Model file for the job. Use its own axes, mm. Round coordinates to 2 decimals unless told otherwise and drop trailing zeros. Loops run counter-clockwise (first coordinate to the right, second up) from the corner with the lowest first, then second, coordinate; pieces in that order, holes last. Notation, with made-up numbers: M -37.5,2 L -31.5,2 A26 ccw -31.5,20 Z; hole C 80,28.5 d8. An arc over 180 degrees is marked long. Use a Markdown table: item, result. Add a question column.
Item 1: Saw through at B-B on y = 150. Write the cut outline in (x, z), then the cut area to 3 significant figures.
Item 2: Saw through at A-A on x = -150. Write the cut outline in (y, z).
Item 3: Wall check: L1, parallel to Y at x = 0, z = 6; L2, parallel to Y at x = 330, z = 2; L3, parallel to X at y = 42, z = 4.25. Give the ranges that are in metal, low to high. Write a range as from..to.
Item 4: Two-plate mould, pull along X, no slides. Class faces 1 (the cylindrical face through (2.222, -10.006, 3.944)), 2 (the flat face through (46, 4, 0)), 3 (the cylindrical face through (-100.301, 103.063, 4.056)): +X half, -X half, draft (parallel to the pull), parting line (faces both ways), or undercut.
Item 5: Pin check, flat tips, straight feed: P1, Ø9, axis at x = 50, y = 210, coming from the +Z side; P2, Ø6, axis at x = -47.5, y = 65.5, coming from the -Z side. Stop position of each tip, or through.
Solid Edge part; units mm, degrees
sketch "Sketch1" plane through (0, 0, 0) normal (0, 0, 1) x (1, 0, 0)
  line L0 (-250, -250) -> (250, -250)
  line L1 (250, -250) -> (250, 250)
  line L2 (250, 250) -> (-250, 250)
  line L3 (-250, 250) -> (-250, -250)
extrude "ProtrusioneEstrusa_1" add sketch "Sketch1" along normal blind 8
hole "Foro_1" at (0, 150, 8) direction (0, 0, -1) diameter 13 end through all
pattern_circular "Pattern1" count 8 over 360 about axis through (0, 0, 8) along (0, 0, -1) of "Foro_1"
sketch "Sketch2" plane through (0, 0, 0) normal (0, 0, -1) x (-1, 0, 0)
  circle A0 centre (0, 0) radius 10.25
extrude "Cutout1" cut sketch "Sketch2" against normal through all
sketch "Sketch3" plane through (0, 0, 8) normal (0, 0, 1) x (-1, 0, 0)
  circle A0 centre (0, 42) radius 2.9585
  circle A1 centre (42, 0) radius 2.9585
  circle A2 centre (0, -42) radius 2.9585
  circle A3 centre (-42, 0) radius 2.9585
extrude "Cutout2" cut sketch "Sketch3" against normal through all
sketch "Sketch4" plane through (0, 0, 8) normal (0, 0, 1) x (1, 0, 0)
  line L0 (250, -250) -> (350, -250)
  line L1 (350, -250) -> (350, 250)
  line L2 (250, 250) -> (350, 250)
  line L3 (250, -250) -> (250, 250)
extrude "Protrusion1" add sketch "Sketch4" against normal up to vertex (8 mm away)
sketch "Sketch5" plane through (50, 0, 8) normal (0, 0, 1) x (1, 0, 0)
  circle A0 centre (-280, -210) radius 5
  circle A1 centre (0, -210) radius 5
  circle A2 centre (280, -210) radius 5
extrude "Cutout3" cut sketch "Sketch5" against normal through all
mirror "Mirror1" about plane through (0, 0, 0) normal (0, -1, 0) of "Cutout3"
sketch "Sketch6" plane through (50, 0, 8) normal (0, 0, 1) x (0, 1, 0)
  arc A0 (-0.2925, -140.7045) -> (2.7075, -140.7045) centre (1.2075, -140.7045) cw
  line L0 (2.7075, -140.7045) -> (2.7075, -147.7045)
  arc A1 (2.7075, -147.7045) -> (-0.2925, -147.7045) centre (1.2075, -147.7045) cw
  line L1 (-0.2925, -140.7045) -> (-0.2925, -147.7045)
  line L2 (-19.4925, -151.0045) -> (-19.4925, -158.0045)
  arc A2 (-19.4925, -158.0045) -> (-22.4925, -158.0045) centre (-20.9925, -158.0045) cw
  line L3 (-22.4925, -151.0045) -> (-22.4925, -158.0045)
  arc A3 (-22.4925, -151.0045) -> (-19.4925, -151.0045) centre (-20.9925, -151.0045) cw
extrude "Cutout5" cut sketch "Sketch6" against normal through all
properties material "Acrylic Plastic (extra strong)"
Entries:
| question | item | result |
|---|---|---|
| 1 | outline | M -250,0 L -6.5,0 L -6.5,8 L -250,8 Z; M 6.5,0 L 350,0 L 350,8 L 6.5,8 Z |
| 1 | area | 4,700 mm2 |
| 2 | outline | M -250,0 L -6.5,0 L -6.5,8 L -250,8 Z; M 6.5,0 L 250,0 L 250,8 L 6.5,8 Z |
| 3 | L1 | -250..-156.5, -143.5..-44.96, -39.04..-10.25, 10.25..39.04, 44.96..143.5, 156.5..250 |
| 3 | L2 | -250..-215, -205..205, 215..250 |
| 3 | L3 | -250..-2.96, 2.96..350 |
| 4 | face 1 | undercut |
| 4 | face 2 | draft |
| 4 | face 3 | undercut |
| 5 | P1 | through |
| 5 | P2 | z = 0 |
